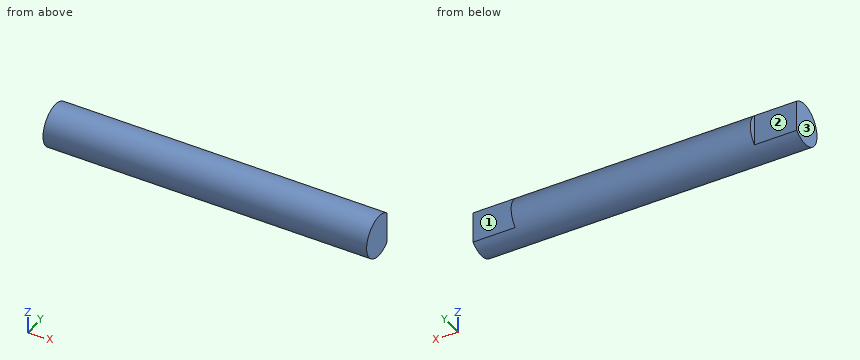
```python
from build123d import *

# Parameters (mm, degrees)
SKETCH2_W          = 46
SKETCH2_H          = 3
CUT_EXTRUDE1_DEPTH = 6
CUT_EXTRUDE2_DEPTH = 6


with BuildPart() as part:
    # Sketch2 → Revolve1 (revolve)
    with BuildSketch(Plane.XY):
        with Locations((23, -1.5)):
            Rectangle(SKETCH2_W, SKETCH2_H)
    revolve(axis=Axis((0, 0, 0), (1, 0, 0)))

    # Sketch3 → Cut-Extrude1 (cut)
    with BuildSketch(Plane(origin=(46, 0, 0), x_dir=(0, 0, -1), z_dir=(1, 0, 0))):
        with BuildLine():
            Line((-2.236067977, 2), (2.236067977, 2))
            ThreePointArc((2.236067977, 2), (0, 3), (-2.236067977, 2))
        make_face()
    extrude(amount=-CUT_EXTRUDE1_DEPTH, mode=Mode.SUBTRACT)

    # Sketch4 → Cut-Extrude2 (cut)
    with BuildSketch(Plane.ZY):
        with BuildLine():
            Line((-2.236067977, 2), (2.236067977, 2))
            ThreePointArc((2.236067977, 2), (0, 3), (-2.236067977, 2))
        make_face()
    extrude(amount=-CUT_EXTRUDE2_DEPTH, mode=Mode.SUBTRACT)


solid = part.part
```
Work out the finished part from the listing and answer in its coordinate system (mm). Face numbers are marked on the shaded views. A direction names the side the tool comes from. Give positions to 0.01 mm unless a question says otherwise; leave off trailing zeros. Write each loop counter-clockwise with the first axis right and the second up, starting at its lowest first coordinate (ties: lowest second). Pieces come first, ordered by that corner, then holes.
(1) Straight lines are drawn through the part: line 1 (X direction, y = 2.35, z = 1.3); line 2 (Z direction, x = 15.5, y = 0.1); line 3 (Z direction, x = 34, y = -2). For each, find the intervals that lie inside material, in ascending order.
Final values:
line 1: x = 6 to 40
line 2: z = -3 to 3
line 3: z = -2.24 to 2.24
(2) The part is cut by section D-D on y = 1.05. Write down the section's boundary in (x, z).
Final values:
outline: (0, -2.81) - (46, -2.81) - (46, 2.81) - (0, 2.81) - close
(3) Flat-ended cylindrical pins translate along their axes: pin 1 Ø0.5 at (y, z) = (2.5, -1) entering from +X; pin 2 Ø3.5 at (x, z) = (3.5, -0.5) entering from +Y; pin 3 Ø2 at (x, y) = (41.5, -1.5) entering from -Z. Find the tip coordinate at first contact, or state that the pin passes through.
Final values:
pin 1: stops at x = 40
pin 2: stops at y = 2
pin 3: stops at z = -2.96
(4) The part is cut by section C-C on z = -1.65. Write down the section's boundary in (x, y), plus the area to 3 significant figures.
Final values:
outline: (0, -2.51) - (46, -2.51) - (46, 2) - (40, 2) - (40, 2.51) - (6, 2.51) - (6, 2) - (0, 2) - close
area: 224 mm2
(5) The part is cut by section B-B on x = 17. Write down the section's boundary in (y, z).
Final values:
outline: circle Ø6 at (0, 0)
(6) The part is cut by section A-A on z = 0. Write down the section's boundary in (x, y).
Final values:
outline: (0, -3) - (46, -3) - (46, 2) - (40, 2) - (40, 3) - (6, 3) - (6, 2) - (0, 2) - close
(7) Which of the six approach directions +Z, -Z, +X, -X, +Y, -Y give full straight-line access (tool end or side, diameter ignored) to the marked faces 1, 2 and 3?
Final values:
face 1: +Z, -Z, +X, +Y
face 2: +Z, -Z, -X, +Y
face 3: +Z, -Z, -X, +Y, -Y
